Can you work these out from the drawing? Everything is in mm from the part's minimum corner. A direction names the side the tool comes from. Round coordinates to 2 decimals unless told otherwise and drop trailing zeros. Order: outer loops, then holes, each group sorted by start corner. A loop starts at its lowest first (then second) coordinate and runs counter-clockwise, first axis right, second up. Notation, with made-up numbers: M -16.75,45 L 25.25,45 A16 cw 25.25,69 Z; hole C 58.25,70 d11. An arc over 180 degrees is marked long. Write item = value, one per line. Start each with the question number.
Item 1: I want a section at D-D, the plane x = 87. List the corners of the cut face in (y, z) for me.
Item 2: I want a section at B-B, the plane x = 304.8. List the corners of the cut face in (y, z) for me.
Item 3: I'm going to push flat-ended pins straight in: P1, Ø4, axis at x = 186.5, z = 181.5, coming from the -Y side; P2, Ø6, axis at y = 183.5, z = 109.5, coming from the -X side; P3, Ø6, axis at x = 249, y = 38.5, coming from the +Z side; P4, Ø24.5, axis at x = 38.1, y = 50.8, coming from the +Z side (3 decimals). Where does each tip first touch, or does it pass through?
Item 4: Please list where these lines run through material, in increasing order: L1, parallel to Y at x = 38.1, z = 10.75; L2, parallel to X at y = 177, z = 11; L3, parallel to Z at x = 170.5, y = 43.5.
Item 5: For the marked faces 5, 6, 7 and 8, which set-ups out of +Z, -Z, +X, -X, +Y, -Y let a thin tool reach every point of the face, with its end or its side?
Item 6: We'd pull the mould along Y, two halves only. Please class the marked faces 1, 2, 3 and 4: pulls with the +Y half, pulls with the -Y half, needs draft (parallel to the pull), parting line crosses it, or undercut.
Item 7: I want a section at A-A, the plane y = 50.8. List the corners of the cut face in (x, z) for me.
Item 8: I want a section at C-C, the plane y = 177.8. List the corners of the cut face in (x, z) for me, plus the area to 3 significant figures.
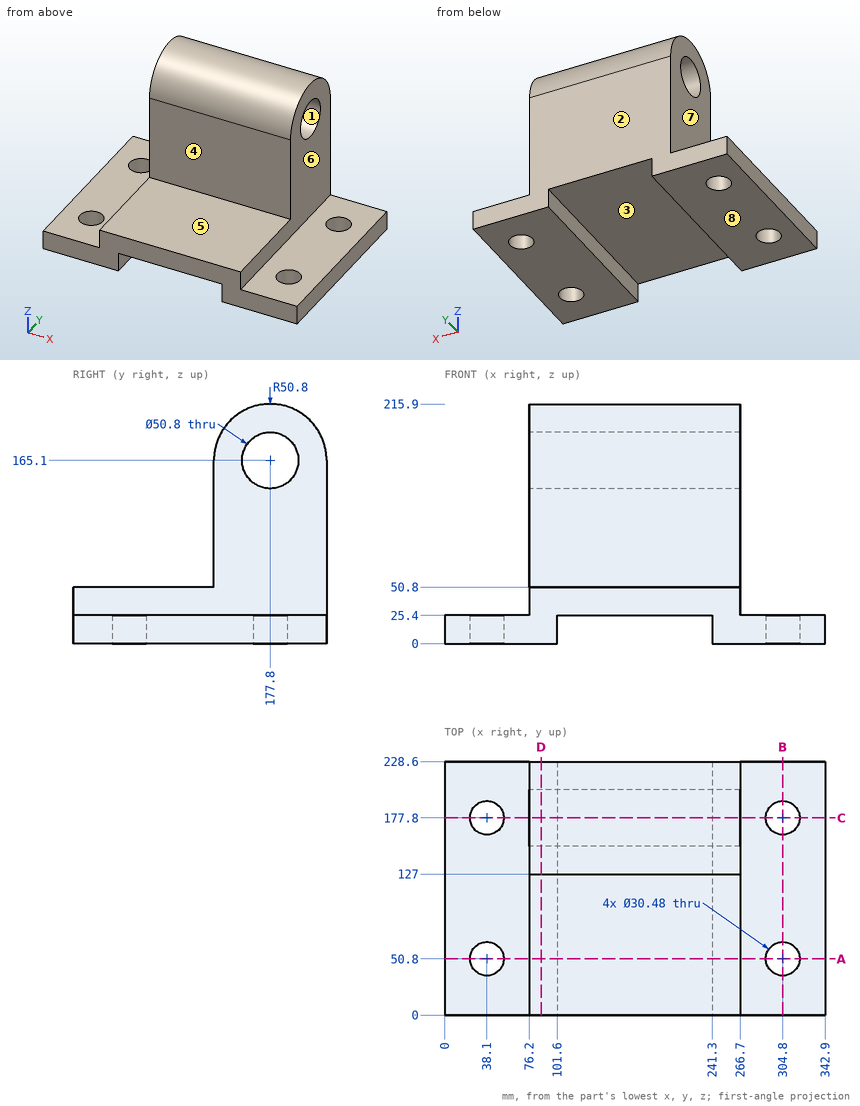
Filled in:
q1.outline = M 0,0 L 228.6,0 L 228.6,165.1 A50.8 ccw 127,165.1 L 127,50.8 L 0,50.8 Z; hole C 177.8,165.1 d50.8
q2.outline = M 0,0 L 35.56,0 L 35.56,25.4 L 0,25.4 Z; M 66.04,0 L 162.56,0 L 162.56,25.4 L 66.04,25.4 Z; M 193.04,0 L 228.6,0 L 228.6,25.4 L 193.04,25.4 Z
q3.P1 = 129.08
q3.P2 = 76.2
q3.P3 = 50.8
q3.P4 = through
q4.L1 = 0 to 35.56, 66.04 to 162.56, 193.04 to 228.6
q4.L2 = 0 to 22.88, 53.32 to 101.6, 241.3 to 289.58, 320.02 to 342.9
q4.L3 = 25.4 to 50.8
q5.face_5 = +Z, +X, -X, -Y
q5.face_6 = +Z, +X, +Y, -Y
q5.face_7 = +Z, -X, +Y, -Y
q5.face_8 = -Z, +X, -X, +Y, -Y
q6.face_1 = undercut
q6.face_2 = pulls with the +Y half
q6.face_3 = needs draft
q6.face_4 = pulls with the -Y half
q7.outline = M 0,0 L 22.86,0 L 22.86,25.4 L 0,25.4 Z; M 53.34,0 L 101.6,0 L 101.6,25.4 L 241.3,25.4 L 241.3,0 L 289.56,0 L 289.56,25.4 L 266.7,25.4 L 266.7,50.8 L 76.2,50.8 L 76.2,25.4 L 53.34,25.4 Z; M 320.04,0 L 342.9,0 L 342.9,25.4 L 320.04,25.4 Z
q8.outline = M 0,0 L 22.86,0 L 22.86,25.4 L 0,25.4 Z; M 53.34,0 L 101.6,0 L 101.6,25.4 L 241.3,25.4 L 241.3,0 L 289.56,0 L 289.56,25.4 L 266.7,25.4 L 266.7,139.7 L 76.2,139.7 L 76.2,25.4 L 53.34,25.4 Z; M 76.2,190.5 L 266.7,190.5 L 266.7,215.9 L 76.2,215.9 Z; M 320.04,0 L 342.9,0 L 342.9,25.4 L 320.04,25.4 Z
q8.area = 30,200 mm^2
